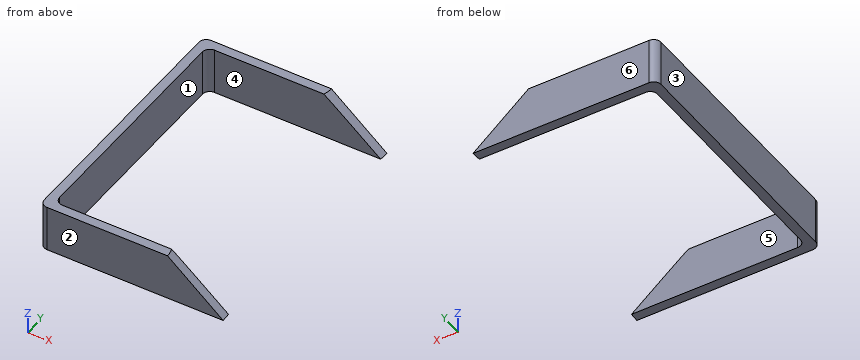
```python
from build123d import *

# Parameters (mm, degrees)
F1_DEPTH     = 3.175
F2_DEPTH     = 19.05
F3_DEPTH     = 3.175
F4_T4_ANGLE  = 359.64
F4_T11_ANGLE = 359.64
F4_T16_ANGLE = 359.64
F4_T18_ANGLE = 359.64
F5_R         = 2.54
F6_W         = 173.444584012
F6_H         = 315.2023479342
F7_DEPTH     = 3.175


# Not quite as in the source:
# - a fillet or chamfer that OpenCascade refuses, or shapes differently, is made with other operations: its cross-section is extruded or revolved along the edge and cut away or added


with BuildPart() as f1:
    # F0 (on Top) → F1 (new body)
    with BuildSketch(Plane.XY):
        with BuildLine():
            Line((-34.925, 44.45), (-28.575, 44.45))
            ThreePointArc((-28.575, 44.45), (-39.4151280605, 48.9401280605), (-34.925, 38.1))
            Line((-34.925, 38.1), (-34.925, 44.45))
        make_face()
        with BuildLine():
            ThreePointArc((6.35, 44.45), (0, 50.8), (-6.35, 44.45))
            Line((-6.35, 44.45), (6.35, 44.45))
        make_face()
        with BuildLine():
            Line((-34.925, -44.45), (-34.925, -38.1))
            ThreePointArc((-34.925, -38.1), (-39.4151280605, -48.9401280605), (-28.575, -44.45))
            Line((-28.575, -44.45), (-34.925, -44.45))
        make_face()
        with BuildLine():
            Line((6.35, -44.45), (-6.35, -44.45))
            ThreePointArc((-6.35, -44.45), (0, -50.8), (6.35, -44.45))
        make_face()
        with BuildLine():
            ThreePointArc((-28.575, 44.45), (-28.7913710031, 42.8064990636), (-29.425738686, 41.275))
            Line((-29.425738686, 41.275), (-5.499261314, 41.275))
            ThreePointArc((-5.499261314, 41.275), (-6.1336289969, 42.8064990636), (-6.35, 44.45))
            Line((-6.35, 44.45), (-28.575, 44.45))
        make_face()
        with BuildLine():
            Line((-5.499261314, -41.275), (-29.425738686, -41.275))
            ThreePointArc((-29.425738686, -41.275), (-28.7913710031, -42.8064990636), (-28.575, -44.45))
            Line((-28.575, -44.45), (-6.35, -44.45))
            ThreePointArc((-6.35, -44.45), (-6.1336289969, -42.8064990636), (-5.499261314, -41.275))
        make_face()
        with BuildLine():
            Line((-31.75, -38.950738686), (-31.75, 38.950738686))
            ThreePointArc((-31.75, 38.950738686), (-33.2814990636, 38.3163710031), (-34.925, 38.1))
            Line((-34.925, 38.1), (-34.925, -38.1))
            ThreePointArc((-34.925, -38.1), (-33.2814990636, -38.3163710031), (-31.75, -38.950738686))
        make_face()
        with BuildLine():
            Line((-31.75, 38.950738686), (-31.75, 41.275))
            Line((-31.75, 41.275), (-29.425738686, 41.275))
            ThreePointArc((-29.425738686, 41.275), (-28.7913710031, 42.8064990636), (-28.575, 44.45))
            Line((-28.575, 44.45), (-34.925, 44.45))
            Line((-34.925, 44.45), (-34.925, 38.1))
            ThreePointArc((-34.925, 38.1), (-33.2814990636, 38.3163710031), (-31.75, 38.950738686))
        make_face()
        with BuildLine():
            ThreePointArc((-6.35, 44.45), (-6.1336289969, 42.8064990636), (-5.499261314, 41.275))
            Line((-5.499261314, 41.275), (5.499261314, 41.275))
            ThreePointArc((5.499261314, 41.275), (6.1336289969, 42.8064990636), (6.35, 44.45))
            Line((6.35, 44.45), (-6.35, 44.45))
        make_face()
        with BuildLine():
            Line((-31.75, -41.275), (-31.75, -38.950738686))
            ThreePointArc((-31.75, -38.950738686), (-33.2814990636, -38.3163710031), (-34.925, -38.1))
            Line((-34.925, -38.1), (-34.925, -44.45))
            Line((-34.925, -44.45), (-28.575, -44.45))
            ThreePointArc((-28.575, -44.45), (-28.7913710031, -42.8064990636), (-29.425738686, -41.275))
            Line((-29.425738686, -41.275), (-31.75, -41.275))
        make_face()
        with BuildLine():
            Line((5.499261314, -41.275), (-5.499261314, -41.275))
            ThreePointArc((-5.499261314, -41.275), (-6.1336289969, -42.8064990636), (-6.35, -44.45))
            Line((-6.35, -44.45), (6.35, -44.45))
            ThreePointArc((6.35, -44.45), (6.1336289969, -42.8064990636), (5.499261314, -41.275))
        make_face()
    extrude(amount=F1_DEPTH)

    # F0 (on Top) → F2 (join)
    with BuildSketch(Plane.XY):
        with BuildLine():
            ThreePointArc((-28.575, 44.45), (-28.7913710031, 42.8064990636), (-29.425738686, 41.275))
            Line((-29.425738686, 41.275), (-5.499261314, 41.275))
            ThreePointArc((-5.499261314, 41.275), (-6.1336289969, 42.8064990636), (-6.35, 44.45))
            Line((-6.35, 44.45), (-28.575, 44.45))
        make_face()
        with BuildLine():
            ThreePointArc((-6.35, 44.45), (-6.1336289969, 42.8064990636), (-5.499261314, 41.275))
            Line((-5.499261314, 41.275), (5.499261314, 41.275))
            ThreePointArc((5.499261314, 41.275), (6.1336289969, 42.8064990636), (6.35, 44.45))
            Line((6.35, 44.45), (-6.35, 44.45))
        make_face()
        with BuildLine():
            Line((-31.75, 38.950738686), (-31.75, 41.275))
            Line((-31.75, 41.275), (-29.425738686, 41.275))
            ThreePointArc((-29.425738686, 41.275), (-28.7913710031, 42.8064990636), (-28.575, 44.45))
            Line((-28.575, 44.45), (-34.925, 44.45))
            Line((-34.925, 44.45), (-34.925, 38.1))
            ThreePointArc((-34.925, 38.1), (-33.2814990636, 38.3163710031), (-31.75, 38.950738686))
        make_face()
        with BuildLine():
            Line((-31.75, -38.950738686), (-31.75, 38.950738686))
            ThreePointArc((-31.75, 38.950738686), (-33.2814990636, 38.3163710031), (-34.925, 38.1))
            Line((-34.925, 38.1), (-34.925, -38.1))
            ThreePointArc((-34.925, -38.1), (-33.2814990636, -38.3163710031), (-31.75, -38.950738686))
        make_face()
        with BuildLine():
            Line((-31.75, -41.275), (-31.75, -38.950738686))
            ThreePointArc((-31.75, -38.950738686), (-33.2814990636, -38.3163710031), (-34.925, -38.1))
            Line((-34.925, -38.1), (-34.925, -44.45))
            Line((-34.925, -44.45), (-28.575, -44.45))
            ThreePointArc((-28.575, -44.45), (-28.7913710031, -42.8064990636), (-29.425738686, -41.275))
            Line((-29.425738686, -41.275), (-31.75, -41.275))
        make_face()
        with BuildLine():
            Line((-5.499261314, -41.275), (-29.425738686, -41.275))
            ThreePointArc((-29.425738686, -41.275), (-28.7913710031, -42.8064990636), (-28.575, -44.45))
            Line((-28.575, -44.45), (-6.35, -44.45))
            ThreePointArc((-6.35, -44.45), (-6.1336289969, -42.8064990636), (-5.499261314, -41.275))
        make_face()
        with BuildLine():
            Line((5.499261314, -41.275), (-5.499261314, -41.275))
            ThreePointArc((-5.499261314, -41.275), (-6.1336289969, -42.8064990636), (-6.35, -44.45))
            Line((-6.35, -44.45), (6.35, -44.45))
            ThreePointArc((6.35, -44.45), (6.1336289969, -42.8064990636), (5.499261314, -41.275))
        make_face()
    extrude(amount=F2_DEPTH)

    # F0 (on Top) → F3 (join)
    with BuildSketch(Plane.XY):
        with BuildLine():
            ThreePointArc((6.35, 44.45), (6.1336289969, 42.8064990636), (5.499261314, 41.275))
            Line((5.499261314, 41.275), (31.75, 41.275))
            Line((31.75, 41.275), (31.75, -41.275))
            Line((31.75, -41.275), (5.499261314, -41.275))
            ThreePointArc((5.499261314, -41.275), (6.1336289969, -42.8064990636), (6.35, -44.45))
            Line((6.35, -44.45), (34.925, -44.45))
            Line((34.925, -44.45), (34.925, 44.45))
            Line((34.925, 44.45), (6.35, 44.45))
        make_face()
        with BuildLine():
            Line((-5.499261314, 41.275), (-29.425738686, 41.275))
            ThreePointArc((-29.425738686, 41.275), (-30.4348719395, 39.9598719395), (-31.75, 38.950738686))
            Line((-31.75, 38.950738686), (-31.75, -38.950738686))
            ThreePointArc((-31.75, -38.950738686), (-30.4348719395, -39.9598719395), (-29.425738686, -41.275))
            Line((-29.425738686, -41.275), (-5.499261314, -41.275))
            ThreePointArc((-5.499261314, -41.275), (0, -38.1), (5.499261314, -41.275))
            Line((5.499261314, -41.275), (31.75, -41.275))
            Line((31.75, -41.275), (31.75, 41.275))
            Line((31.75, 41.275), (5.499261314, 41.275))
            ThreePointArc((5.499261314, 41.275), (0, 38.1), (-5.499261314, 41.275))
        make_face()
        with BuildLine():
            Line((5.499261314, 41.275), (-5.499261314, 41.275))
            ThreePointArc((-5.499261314, 41.275), (0, 38.1), (5.499261314, 41.275))
        make_face()
        with BuildLine():
            Line((-29.425738686, 41.275), (-31.75, 41.275))
            Line((-31.75, 41.275), (-31.75, 38.950738686))
            ThreePointArc((-31.75, 38.950738686), (-30.4348719395, 39.9598719395), (-29.425738686, 41.275))
        make_face()
        with BuildLine():
            ThreePointArc((5.499261314, -41.275), (0, -38.1), (-5.499261314, -41.275))
            Line((-5.499261314, -41.275), (5.499261314, -41.275))
        make_face()
        with BuildLine():
            ThreePointArc((-29.425738686, -41.275), (-30.4348719395, -39.9598719395), (-31.75, -38.950738686))
            Line((-31.75, -38.950738686), (-31.75, -41.275))
            Line((-31.75, -41.275), (-29.425738686, -41.275))
        make_face()
    extrude(amount=F3_DEPTH)

    # F4: chamfer of 17.78 x 21.1893788763 on 4 edges, made by hand


with BuildPart() as f4_tool2:
    # F4_s3 → F4_t4 (revolve)
    with BuildSketch(Plane(origin=(-7.9045602021, -1.4531788711, 0), x_dir=(0, 0, 1), z_dir=(-0.983517952, -0.1808105031, 0))):
        Polygon((3.175, -16.1779940912), (20.955, -37.3673729675), (3.175, -37.3673729675), align=None)
    revolve(axis=Axis((0, -44.45, 3.175), (0, 0, -1)), revolution_arc=F4_T4_ANGLE)

    split(bisect_by=Plane.XY.offset(19.05), keep=Keep.BOTTOM)

    split(bisect_by=Plane.XZ.offset(44.45), keep=Keep.BOTTOM)

    split(bisect_by=Plane.XZ.offset(41.275), keep=Keep.TOP)


with BuildPart() as f1_1:
    add(f1.part)

    # F4_t1: union F4_tool2
    add(f4_tool2.part)


with BuildPart() as f4_tool9:
    # F4_s10 → F4_t11 (revolve)
    with BuildSketch(Plane(origin=(-8.164955624, 1.5541479455, 0), x_dir=(0, 0, 1), z_dir=(0.9823624798, -0.186986519, 0))):
        Polygon((20.955, -37.3160122271), (3.175, -16.1266333508), (3.175, -37.3160122271), align=None)
    revolve(axis=Axis((0, 44.45, 3.175), (0, 0, -1)), revolution_arc=F4_T11_ANGLE)

    split(bisect_by=Plane.XZ.offset(-44.45), keep=Keep.TOP)

    split(bisect_by=Plane.XY.offset(19.05), keep=Keep.BOTTOM)

    split(bisect_by=Plane.XZ.offset(-41.275), keep=Keep.BOTTOM)


with BuildPart() as f1_2:
    add(f1_1.part)

    # F4_t8: union F4_tool9
    add(f4_tool9.part)

    # F4_s15 → F4_t16 (revolve, cut)
    with BuildSketch(Plane(origin=(-0.1396428746, -0.0004387025, 0), x_dir=(0, 0, 1), z_dir=(0.9999950652, 0.0031415875, 0))):
        Polygon((-14.605, 38.0997806482), (-9.276717342, 44.4497806482), (3.175, 44.4497806482), (3.175, 38.0997806482), align=None)
    revolve(axis=Axis((0, -44.45, 3.175), (0, 0, 1)), revolution_arc=F4_T16_ANGLE, mode=Mode.SUBTRACT)

    # F4_s17 → F4_t18 (revolve, cut)
    with BuildSketch(Plane(origin=(0.1396428746, 0.0004387025, 0), x_dir=(0, 0, 1), z_dir=(-0.9999950652, -0.0031415875, 0))):
        Polygon((-14.605, 38.0997806482), (-9.276717342, 44.4497806482), (3.175, 44.4497806482), (3.175, 38.0997806482), align=None)
    revolve(axis=Axis((0, 44.45, 3.175), (0, 0, 1)), revolution_arc=F4_T18_ANGLE, mode=Mode.SUBTRACT)

    # F5
    f5_edges = [f1_2.edges().sort_by_distance(p)[0] for p in [
        (-31.75, 41.275, 11.1125),
        (-31.75, -41.275, 11.1125),
        (-34.925, -44.45, 11.1125),
        (-34.925, 44.45, 11.1125),
    ]]
    fillet(f5_edges, radius=F5_R)

    # F6 (on Top) → F7 (cut)
    with BuildSketch(Plane.XY):
        with Locations((-10.1288706064, 37.9523970187)):
            Rectangle(F6_W, F6_H)
    extrude(amount=F7_DEPTH, mode=Mode.SUBTRACT)


solid = f1_2.part
```
Could you check a few things on this model? Use its own coordinates, in mm. Face numbers are marked on the shaded views. A direction names the side the tool comes from. Coordinates: 2 decimals unless noted, no trailing zeros. Write each loop counter-clockwise with the first axis right and the second up, starting at its lowest first coordinate (ties: lowest second). Pieces come first, ordered by that corner, then holes. Notation, with made-up numbers: (25.25, 16.5) -> (40.25, 16.5) arc R20 cw to (40.25, 41.5) -> close; hole circle Ø10 at (77.5, -16). An arc over 180 degrees is marked (long way). Return JSON: item names as keys, results as strings.
(1) Imagine slicing it at C-C, the plane y = -28. Please give me the cut outline in (x, z) (3 decimals).
Numbers:
{"outline": "(-34.925, 3.175) -> (-31.75, 3.175) -> (-31.75, 19.05) -> (-34.925, 19.05) -> close"}
(2) Imagine slicing it at B-B, the plane z = 13.75. Please give me the cut outline in (x, y) (3 decimals).
Numbers:
{"outline": "(-34.925, -41.91) arc R2.54 ccw to (-32.385, -44.45) -> (14.937, -44.45) arc R14.937 ccw to (14.595, -41.275) -> (-29.21, -41.275) arc R2.54 cw to (-31.75, -38.735) -> (-31.75, 38.735) arc R2.54 cw to (-29.21, 41.275) -> (14.595, 41.275) arc R14.937 ccw to (14.937, 44.45) -> (-32.385, 44.45) arc R2.54 ccw to (-34.925, 41.91) -> close"}
(3) Which directions (+Z, -Z, +X, -X, +Y, -Y) give clear straight access to the entire face, cutting with the end or side of a thin tool? Please do the marked faces 5 and 6.
Numbers:
{"face 5": "+Z, -Z, +X", "face 6": "+Z, -Z, +X, -X, +Y"}
(4) I'm going to push a flat-ended pin straight in: pin 1 (5 mm diameter, centred on y = 11.5, z = 8, fed in from +X). Where does the tip first touch, or does it pass through?
Numbers:
{"pin 1": "stops at x = -31.75"}
(5) Imagine slicing it at A-A, the plane x = 6. Please give me the cut outline in (y, z) (3 decimals).
Numbers:
{"outline": "(-44.45, 3.175) -> (-41.275, 3.175) -> (-41.275, 19.05) -> (-44.45, 19.05) -> close; (41.275, 3.175) -> (44.45, 3.175) -> (44.45, 19.05) -> (41.275, 19.05) -> close"}
(6) We'd pull the mould along Y, two halves only. Please class the marked faces 1, 2, 3 and 4: +Y half, -Y half, draft (parallel to the pull), parting line (faces both ways), or undercut.
Numbers:
{"face 1": "undercut", "face 2": "-Y half", "face 3": "draft", "face 4": "undercut"}
(7) I need wall thicknesses on L1, parallel to Y at x = -23, z = 14.5 (3 decimals); L2, parallel to X at y = 29, z = 5 (3 decimals). Which ranges of each line are inside material? Lowest first, please.
Numbers:
{"L1": "y = -44.45 to -41.275, 41.275 to 44.45", "L2": "x = -34.925 to -31.75"}
(8) Imagine slicing it at D-D, the plane z = 9.75. Please give me the cut outline in (x, y) (3 decimals).
Numbers:
{"outline": "(-34.925, -41.91) arc R2.54 ccw to (-32.385, -44.45) -> (19.704, -44.45) arc R19.704 ccw to (19.446, -41.275) -> (-29.21, -41.275) arc R2.54 cw to (-31.75, -38.735) -> (-31.75, 38.735) arc R2.54 cw to (-29.21, 41.275) -> (19.446, 41.275) arc R19.704 ccw to (19.704, 44.45) -> (-32.385, 44.45) arc R2.54 ccw to (-34.925, 41.91) -> close"}
